Design review of the part shown in the three views and the two pictorial views. Dimensions are in mm from the part's minimum x, y and z. A direction names the side the tool comes from. Give positions to 0.01 mm unless a question says otherwise; leave off trailing zeros. Write each loop counter-clockwise with the first axis right and the second up, starting at its lowest first coordinate (ties: lowest second). Pieces come first, ordered by that corner, then holes.
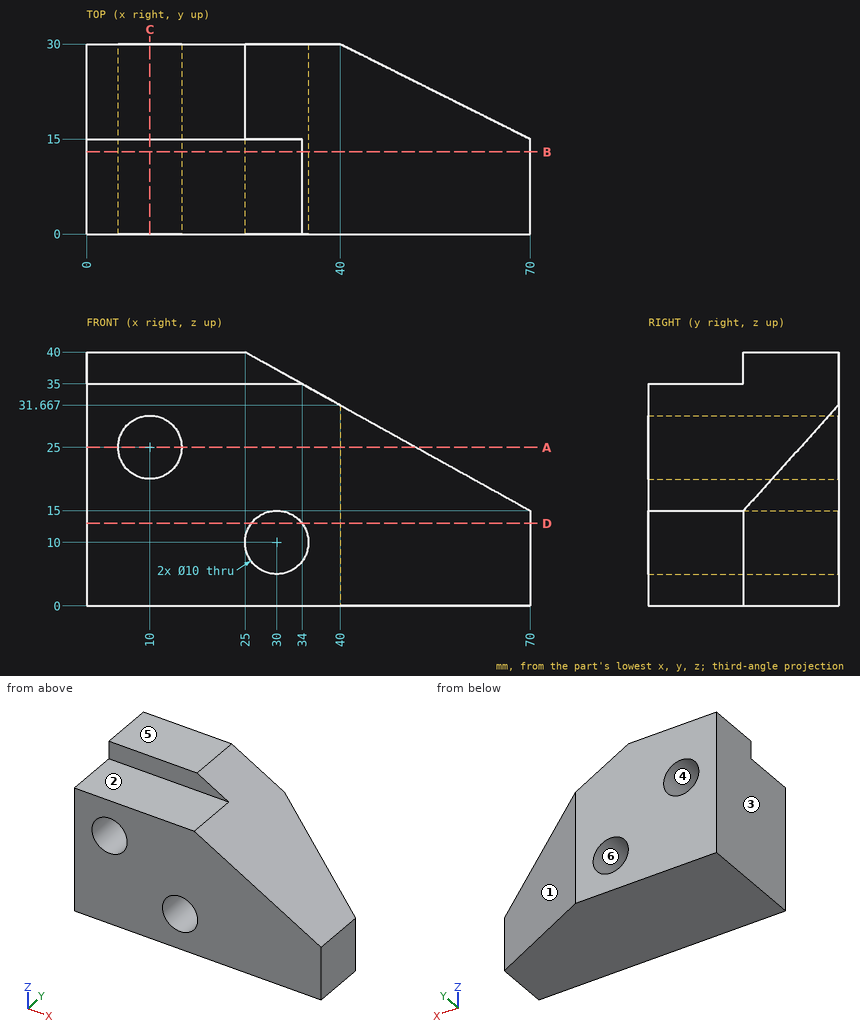
(1) Consider section A-A, the plane z = 25. Give the boundary of the cut face in (x, y), then the cut area to 3 significant figures.
Resolved:
outline: (0, 0) - (5, 0) - (5, 30) - (0, 30) - close; (15, 0) - (52, 0) - (52, 24) - (40, 30) - (15, 30) - close
area: 1,220 mm2
(2) Mouldability with a two-part tool opening along Z and no side actions: class the marked faces 3, 4, 5 and 6 as pulls with the +Z half, pulls with the -Z half, needs draft (parallel to the pull), parting line crosses it, or undercut.
Resolved:
face 3: needs draft
face 4: undercut
face 5: pulls with the +Z half
face 6: undercut
(3) Clearance check with flat-ended pins moving along their axes: P1, Ø6, axis at x = 30, z = 10, coming from the +Y side; P2, Ø4, axis at x = 38, y = 9, coming from the +Z side; P3, Ø7.5, axis at x = 24, y = 6, coming from the +Z side; P4, Ø4, axis at x = 42.5, y = 9, coming from the +Z side. State where each tip first meets the part, or that it passes through.
Resolved:
P1: passes through
P2: stops at z = 33.89
P3: stops at z = 35
P4: stops at z = 31.39
(4) Consider section C-C, the plane x = 10. Give the boundary of the cut face in (y, z).
Resolved:
outline: (0, 0) - (30, 0) - (30, 20) - (0, 20) - close; (0, 30) - (30, 30) - (30, 40) - (15, 40) - (15, 35) - (0, 35) - close
(5) Consider section D-D, the plane z = 13. Give the boundary of the cut face in (x, y).
Resolved:
outline: (0, 0) - (26, 0) - (26, 30) - (0, 30) - close; (34, 0) - (70, 0) - (70, 15) - (40, 30) - (34, 30) - close
(6) Consider section B-B, the plane y = 13. Give the boundary of the cut face in (x, z), then the cut area to 3 significant figures.
Resolved:
outline: (0, 0) - (70, 0) - (70, 15) - (34, 35) - (0, 35) - close; hole circle Ø10 at (10, 25); hole circle Ø10 at (30, 10)
area: 1,930 mm2
(7) To check wall thickness, follow L1, parallel to Z at x = 30, y = 9; L2, parallel to Z at x = 10, y = 7.5; L3, parallel to X at y = 27, z = 20.5. State the ranges of each line that lie inside material, in increasing order.
Resolved:
L1: z = 0 to 5, 15 to 35
L2: z = 0 to 20, 30 to 35
L3: x = 0 to 7.82, 12.18 to 46
(8) Tool access review of the marked faces 1 and 2: name each direction out of +Z, -Z, +X, -X, +Y, -Y from which nothing blocks a thin tool from reaching the whole face with its end or side.
Resolved:
face 1: +Z, -Z, +X, +Y
face 2: +Z, +X, -X, -Y
